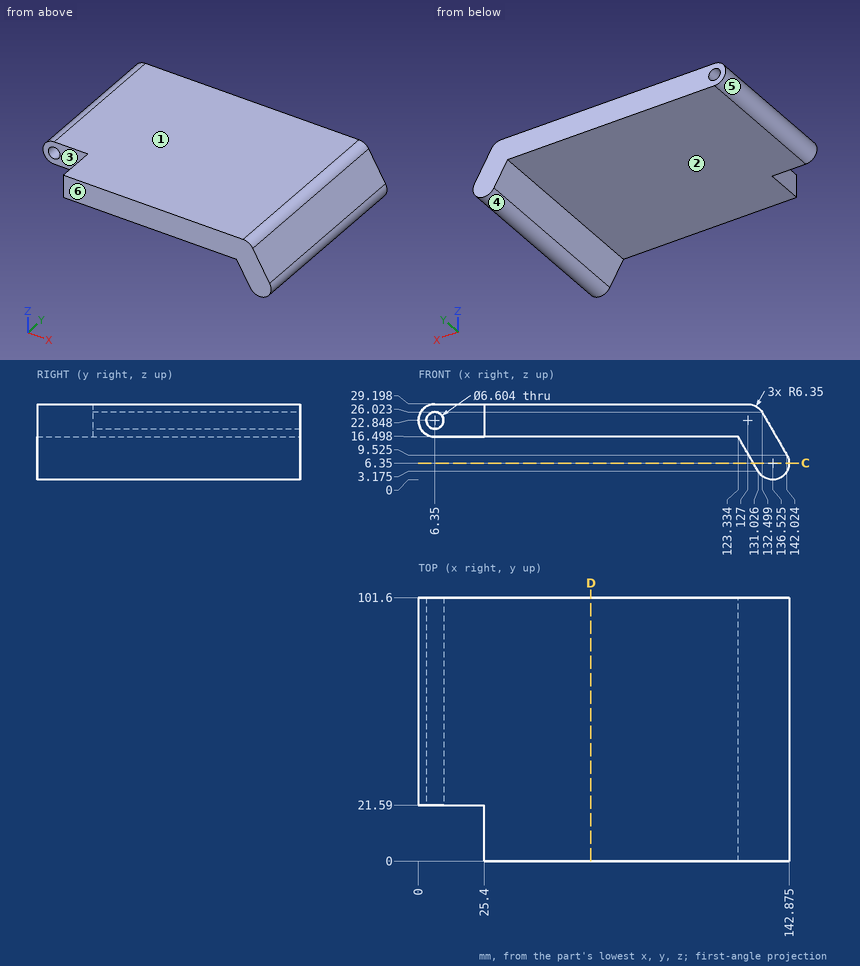
Source: three-view drawing plus pictorial views. Frame: mm from the lowest corner of the part. A direction names the side the tool comes from. Round coordinates to 2 decimals unless told otherwise and drop trailing zeros. Order: outer loops, then holes, each group sorted by start corner. A loop starts at its lowest first (then second) coordinate and runs counter-clockwise, first axis right, second up. Notation, with made-up numbers: (81.5, 20) - (120.5, 20) arc R23 cw to (120.5, 50) - close; hole circle Ø5 at (59.25, 27). An arc over 180 degrees is marked (long way). Answer in a Markdown table with one row per item.
Item 1: Section query D-D (x = 66.5). Return the cut outline in (y, z).
Model answer:
| item | result |
|---|---|
| outline | (0, 16.5) - (101.6, 16.5) - (101.6, 29.2) - (0, 29.2) - close |
Item 2: Reachability of the marked faces 1, 2 and 3 from +Z, -Z, +X, -X, +Y, -Y: full face, straight path, thin tool, end or side. Return the list, or none.
Model answer:
| item | result |
|---|---|
| face 1 | +Z, +X, -X, +Y, -Y |
| face 2 | -Z, -X, +Y, -Y |
| face 3 | +Z, -Z, -X, -Y |
Item 3: Pin query (flat end, axial travel): pin 1 (6.5 mm diameter, centred on y = 16, z = 26, fed in from -X); pin 2 (2 mm diameter, centred on x = 37.5, y = 74, fed in from -Z); pin 3 (4 mm diameter, centred on y = 24, z = 19.5, fed in from -X) (1 decimal). Return the tip coordinate at first contact, or that it passes through.
Model answer:
| item | result |
|---|---|
| pin 1 | stops at x = 25.4 |
| pin 2 | stops at z = 16.5 |
| pin 3 | stops at x = 0.1 |
Item 4: Section query C-C (z = 6.35). Return the cut outline in (x, y) (1 decimal), then the cut area to 3 significant figures.
Model answer:
| item | result |
|---|---|
| outline | (129.2, 0) - (142.9, 0) - (142.9, 101.6) - (129.2, 101.6) - close |
| area | 1,390 mm² |
Item 5: Mould query, pull axis X, two halves, no side actions, for the marked faces 4, 5 and 6. Classes: released by +X, released by -X, zero draft, split by the parting line, or undercut.
Model answer:
| item | result |
|---|---|
| face 4 | split by the parting line |
| face 5 | released by -X |
| face 6 | zero draft |
Item 6: Line query: line 1 (Z direction, x = 6.35, y = 41.5); line 2 (Z direction, x = 6, y = 63) (1 decimal); line 3 (Z direction, x = 62.5, y = 19.5). Output: solid intervals per line, ascending.
Model answer:
| item | result |
|---|---|
| line 1 | z = 16.5 to 19.55, 26.15 to 29.2 |
| line 2 | z = 16.5 to 19.6, 26.1 to 29.2 |
| line 3 | z = 16.5 to 29.2 |
